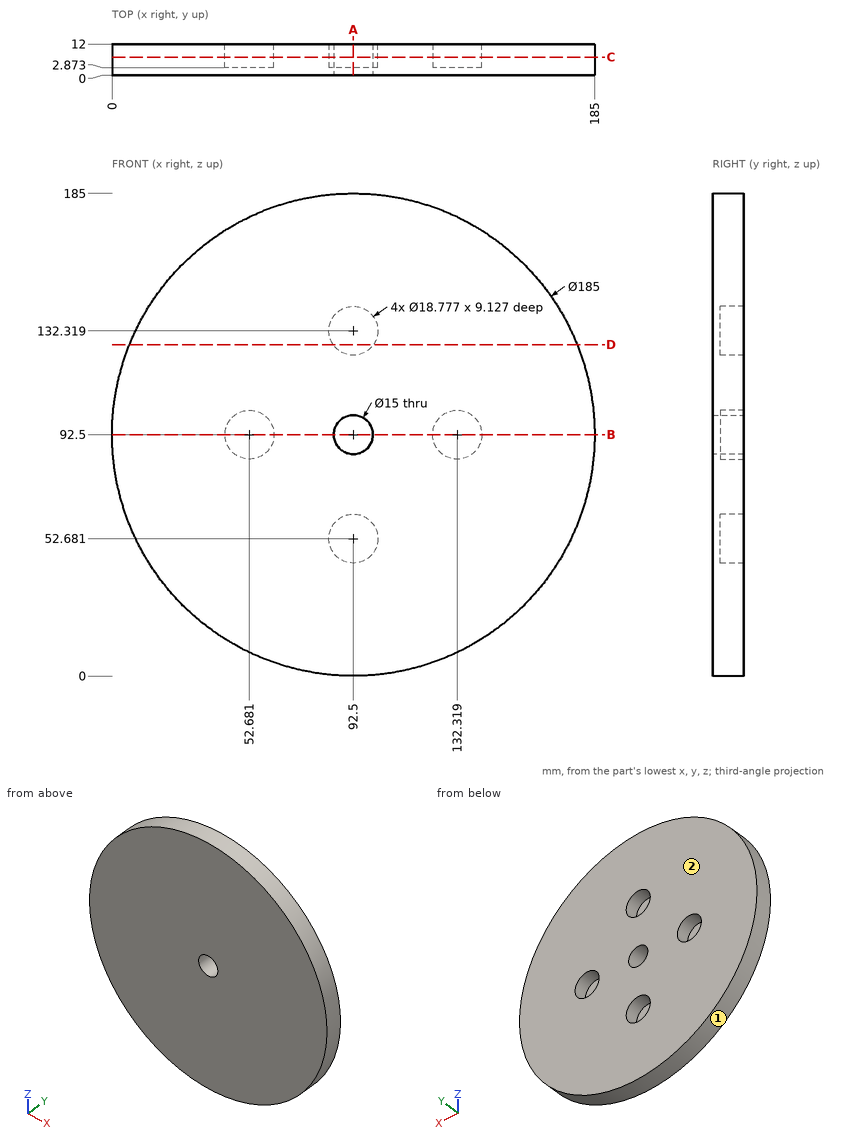
Verification items for this drawing (mm, ordinates from the low corner). Round coordinates to 2 decimals unless told otherwise and drop trailing zeros. Order: outer loops, then holes, each group sorted by start corner. A loop starts at its lowest first (then second) coordinate and runs counter-clockwise, first axis right, second up.
1) Depth check by flat-ended pin: pin 1 (24 mm diameter, centred on x = 92.5, z = 92.5, fed in from -Y); pin 2 (15 mm diameter, centred on x = 92.5, z = 52.68, fed in from +Y); pin 3 (2 mm diameter, centred on x = 45, y = 3.5, fed in from +Z); pin 4 (1 mm diameter, centred on y = 3.5, z = 135.5, fed in from +X). Enter the tip coordinate at first touch or a pass-through.
Geometry says:
pin 1: stops at y = 0
pin 2: stops at y = 2.87
pin 3: stops at z = 172.46
pin 4: stops at x = 174.66
2) Cross-section at C-C, the plane y = 7. Record the cut outline in (x, z), plus the area to 3 significant figures.
Geometry says:
outline: circle Ø185 at (92.5, 92.5); hole circle Ø18.78 at (52.68, 92.5); hole circle Ø18.78 at (92.5, 52.68); hole circle Ø18.78 at (92.5, 132.32); hole circle Ø15 at (92.5, 92.5); hole circle Ø18.78 at (132.32, 92.5)
area: 25,600 mm2
3) Cross-section at A-A, the plane x = 92.5. Record the cut outline in (y, z).
Geometry says:
outline: (0, 0) - (12, 0) - (12, 43.29) - (2.87, 43.29) - (2.87, 62.07) - (12, 62.07) - (12, 85) - (0, 85) - close; (0, 100) - (12, 100) - (12, 122.93) - (2.87, 122.93) - (2.87, 141.71) - (12, 141.71) - (12, 185) - (0, 185) - close
4) Draft check along X on the marked faces 1 and 2. Enter one of: +X half, -X half, draft (parallel to the pull), parting line (faces both ways), or undercut.
Geometry says:
face 1: parting line
face 2: draft
5) Cross-section at B-B, the plane z = 92.5. Record the cut outline in (x, y).
Geometry says:
outline: (0, 0) - (85, 0) - (85, 12) - (62.07, 12) - (62.07, 2.87) - (43.29, 2.87) - (43.29, 12) - (0, 12) - close; (100, 0) - (185, 0) - (185, 12) - (141.71, 12) - (141.71, 2.87) - (122.93, 2.87) - (122.93, 12) - (100, 12) - close
6) Material ranges on line 1 (X direction, y = 7.75, z = 92.5); line 2 (Z direction, x = 86.5, y = 8.5) (1 decimal); line 3 (Z direction, x = 132.5, y = 11.25) (1 decimal), recorded low to high.
Geometry says:
line 1: x = 0 to 43.29, 62.07 to 85, 100 to 122.93, 141.71 to 185
line 2: z = 0.2 to 45.5, 59.9 to 88, 97 to 125.1, 139.5 to 184.8
line 3: z = 9.1 to 83.1, 101.9 to 175.9
7) Cross-section at D-D, the plane z = 127. Record the cut outline in (x, y) (1 decimal), plus the area to 3 significant figures.
Geometry says:
outline: (6.7, 0) - (178.3, 0) - (178.3, 12) - (100.2, 12) - (100.2, 2.9) - (84.8, 2.9) - (84.8, 12) - (6.7, 12) - close
area: 1,920 mm2
